Geometry: see drawing. Coordinates: mm, zero at the bounding-box minimum. Give positions to 0.01 mm unless a question says otherwise; leave off trailing zeros. Loops run counter-clockwise (first coordinate to the right, second up) from the corner with the lowest first, then second, coordinate; pieces in that order, holes last. Notation, with made-up numbers: (74, 20.5) -> (129, 20.5) arc R19 ccw to (129, 50.5) -> close; hole circle Ø11 at (-14.5, 10). An arc over 180 degrees is marked (long way). Return JSON: item names as keys, results as strings. Group by question number.
(1) Pin query (flat end, axial travel): pin 1 (1.5 mm diameter, centred on x = 3.5, z = 2.5, fed in from +Y); pin 2 (3.5 mm diameter, centred on x = 4.5, y = 4.5, fed in from -Z). Return the tip coordinate at first contact, or that it passes through.
(2) Draft query along X for the marked faces 1, 2 and 3. Return one class per face: released by +X, released by -X, zero draft, split by the parting line, or undercut.
(3) Cut plane D-D on y = 11.75. Return loops of the section in (x, z), then the cut area to 3 significant figures.
(4) Cut plane B-B on y = 3.25. Return loops of the section in (x, z).
(5) Cut plane A-A on x = 14.5. Return loops of the section in (y, z), then the cut area to 3 significant figures.
(6) Ray query, line 1 (Y direction, x = 14.5, z = 0.6); line 2 (X direction, y = 14.75, z = 1.1); line 3 (Y direction, x = 4.5, z = 2.25). Return the intervals inside material, ascending. Write a range as from..to.
(7) Cut plane C-C on z = 1.8. Return loops of the section in (x, y), then the cut area to 3 significant figures.
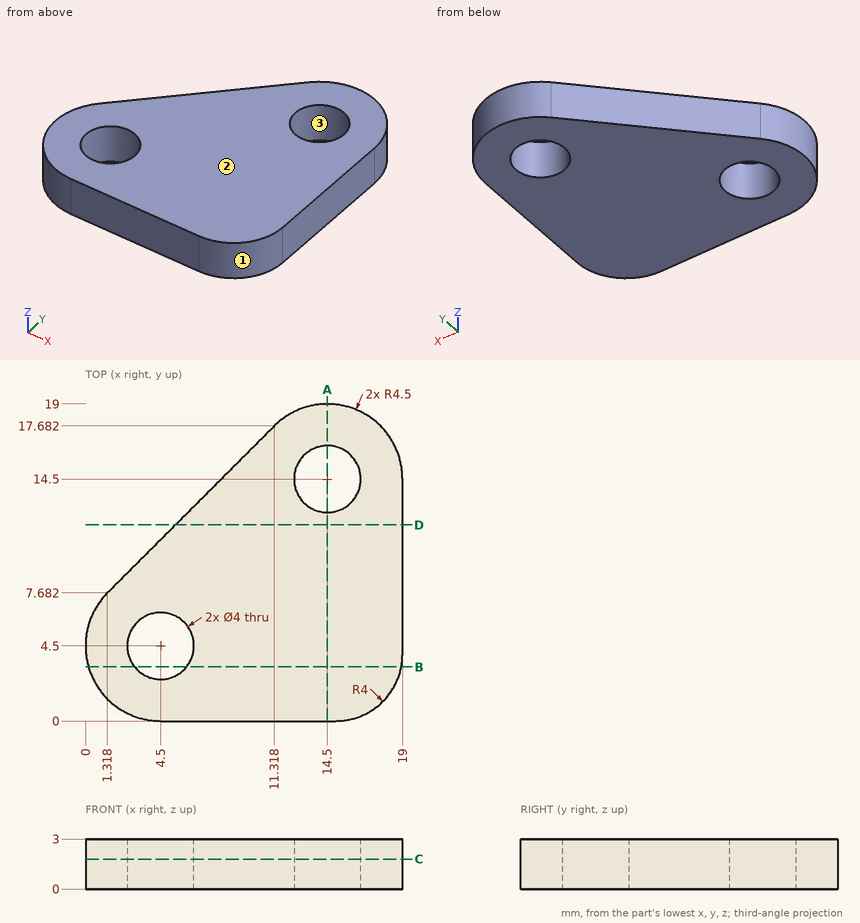
Answers:
{
 "1": {"pin 1": "y = 10.61", "pin 2": "through"},
 "2": {"face 1": "released by +X", "face 2": "zero draft", "face 3": "undercut"},
 "3": {"outline": "(5.39, 0) -> (19, 0) -> (19, 3) -> (5.39, 3) -> close", "area": "40.8 mm²"},
 "4": {"outline": "(0.18, 0) -> (2.94, 0) -> (2.94, 3) -> (0.18, 3) -> close; (6.06, 0) -> (18.93, 0) -> (18.93, 3) -> (6.06, 3) -> close"},
 "5": {"outline": "(0, 0) -> (12.5, 0) -> (12.5, 3) -> (0, 3) -> close; (16.5, 0) -> (19, 0) -> (19, 3) -> (16.5, 3) -> close", "area": "45.0 mm²"},
 "6": {"line 1": "0..12.5, 16.5..19", "line 2": "8.39..12.52, 16.48..18.99", "line 3": "0..2.5, 6.5..10.86"},
 "7": {"outline": "(1.32, 7.68) arc R4.5 ccw to (4.5, 0) -> (15, 0) arc R4 ccw to (19, 4) -> (19, 14.5) arc R4.5 ccw to (11.32, 17.68) -> close; hole circle Ø4 at (4.5, 4.5); hole circle Ø4 at (14.5, 14.5)", "area": "243 mm²"}
}
